Verification items for the finished model (mm, model axes). Face numbers are marked on the shaded views. Coordinates: 2 decimals unless noted, no trailing zeros. Write each loop counter-clockwise with the first axis right and the second up, starting at its lowest first coordinate (ties: lowest second). Pieces come first, ordered by that corner, then holes. Notation, with made-up numbers: M 39.5,78.25 L 56.5,78.25 A22 ccw 56.5,86.25 Z; hole C -24,-33 d2. An arc over 180 degrees is marked long. One line per item, written item: value.
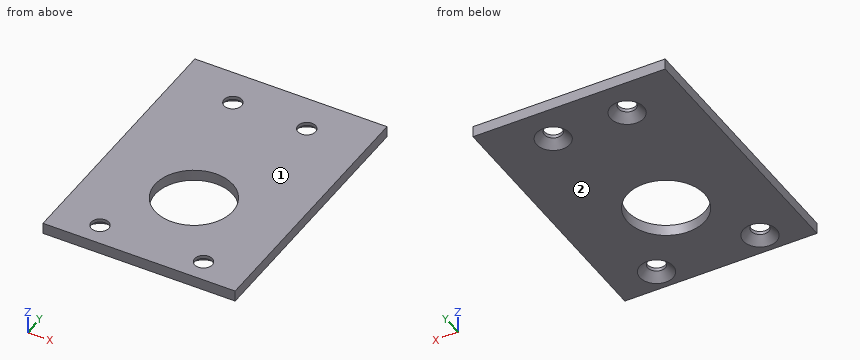
Autodesk Inventor part; units mm, degrees
ref_plane "YZ Plane" through (0, 0, 0) normal (1, 0, 0) x (0, 1, 0)
ref_plane "XZ Plane" through (0, 0, 0) normal (0, 1, 0) x (-1, 0, 0)
ref_plane "XY Plane" through (0, 0, 0) normal (0, 0, 1) x (1, 0, 0)
sketch "Skizze1" plane through (0, 0, 0) normal (0, 0, 1) x (1, 0, 0)
  line L0 (-5.2, 0) -> (31.2, 0)
  line L1 (0, -7.2) -> (0, 43.2)
  line L2 (0, 0) -> (26, 0)
  line L3 (26, 0) -> (26, 36)
  line L4 (26, 36) -> (0, 36)
  line L5 (0, 36) -> (0, 0)
  dimension "d0" = 36
  dimension "d1" = 26
extrude "Extrusion1" add sketch "Skizze1" along normal blind 1.5
sketch "Skizze2" plane through (0, 0, 0) normal (0, 0, -1) x (-1, 0, 0)
  circle A0 centre (-13, 13) radius 4.8
hole "Bohrung1" at (13, 13, 0) direction (0, 0, 1) diameter 10.5 end through all
sketch "Skizze3" plane through (0, 0, 0) normal (0, 0, -1) x (-1, 0, 0)
  line L0 (0, 0) -> (-26, 0)
  line L1 (-26, 36) -> (0, 36)
  line L2 (-20, 31) -> (-6, 31)
  line L3 (-6, 31) -> (-6, 3)
  line L4 (-6, 3) -> (-20, 3)
  line L5 (-20, 3) -> (-20, 31)
  line L6 (-13, 36) -> (-13, 0)
  point P0 (-18, 31)
  point P1 (-8, 31)
  dimension "d11" = 28
  dimension "d12" = 14
  dimension "d20" = 3
  dimension "d21" = 10
hole "Bohrung2" at (18, 31, 0) at (8, 31, 0) at (20, 3, 0) at (6, 3, 0) direction (0, 0, 1) diameter 2.4 end through all countersink diameter 4.5 countersink angle 90
properties part number "13_1087_021"
Item 1: Draft check along Z on the marked faces 1 and 2. Enter one of: released by +Z, released by -Z, zero draft, split by the parting line, or undercut.
The answers:
face 1: released by +Z
face 2: released by -Z
Item 2: Cross-section at A-A, the plane x = 13. Enter the section's corners in (y, z).
The answers:
outline: M 0,0 L 7.75,0 L 7.75,1.5 L 0,1.5 Z; M 18.25,0 L 36,0 L 36,1.5 L 18.25,1.5 Z
Item 3: Cross-section at B-B, the plane y = 31. Enter the section's corners in (x, z), and give its area (3 significant figures).
The answers:
outline: M 0,0 L 5.75,0 L 6.8,1.05 L 6.8,1.5 L 0,1.5 Z; M 9.2,1.05 L 10.25,0 L 15.75,0 L 16.8,1.05 L 16.8,1.5 L 9.2,1.5 Z; M 19.2,1.05 L 20.25,0 L 26,0 L 26,1.5 L 19.2,1.5 Z
area: 29.6 mm²
Item 4: Cross-section at C-C, the plane z = 0.8. Enter the section's corners in (x, y).
The answers:
outline: M 0,0 L 26,0 L 26,36 L 0,36 Z; hole C 6,3 d2.9; hole C 8,31 d2.9; hole C 13,13 d10.5; hole C 18,31 d2.9; hole C 20,3 d2.9
Item 5: Go/stop test with flat-tipped pins: P1, Ø9.5, axis at x = 13, y = 13, coming from the -Z side; P2, Ø4, axis at x = 8, y = 31, coming from the -Z side. Record where each tip stops, or that it passes through.
The answers:
P1: passes through
P2: stops at z = 0.25
Item 6: Scan lines: line 1 (X direction, y = 31, z = 1.3); line 2 (X direction, y = 3, z = 1.3); line 3 (Y direction, x = 13, z = 1). Record each from-to range of solid material in increasing order.
The answers:
line 1: x = 0 to 6.8, 9.2 to 16.8, 19.2 to 26
line 2: x = 0 to 4.8, 7.2 to 18.8, 21.2 to 26
line 3: y = 0 to 7.75, 18.25 to 36
Item 7: Cross-section at D-D, the plane y = 13. Enter the section's corners in (x, z), and give its area (4 significant figures).
The answers:
outline: M 0,0 L 7.75,0 L 7.75,1.5 L 0,1.5 Z; M 18.25,0 L 26,0 L 26,1.5 L 18.25,1.5 Z
area: 23.25 mm²
